Autodesk Inventor part; units mm, degrees
ref_plane "YZ Plane" through (0, 0, 0) normal (1, 0, 0) x (0, 1, 0)
ref_plane "XZ Plane" through (0, 0, 0) normal (0, 1, 0) x (-1, 0, 0)
ref_plane "XY Plane" through (0, 0, 0) normal (0, 0, 1) x (1, 0, 0)
sketch "Sketch1" plane through (0, 0, 0) normal (0, 0, 1) x (1, 0, 0)
  line L0 (0, 0) -> (0, -57.15) construction
  line L1 (0, 0) -> (-53.8815, -53.8815) construction
  line L2 (12.7, 3.175) -> (-14.7855, 3.175)
  line L3 (-14.7855, 3.175) -> (-62.8618, -44.9013)
  line L4 (-62.8618, -44.9013) -> (-44.9013, -62.8618)
  line L5 (-44.9013, -62.8618) -> (-12.7, -30.6605)
  line L6 (-12.7, -30.6605) -> (-12.7, -57.15)
  line L7 (-12.7, -57.15) -> (12.7, -57.15)
  line L8 (12.7, -57.15) -> (12.7, 3.175)
  dimension "d0" = 45
  dimension "d1" = 57.15
  dimension "d2" = 76.2
  dimension "d3" = 3.175
  dimension "d4" = 25.4
  dimension "d5" = 25.4
extrude "Extrusion1" add sketch "Sketch1" against normal blind 6.35
sketch "Sketch2" plane through (0, 0, 0) normal (0, 0, 1) x (1, 0, 0)
  line L0 (-44.9013, -62.8618) -> (-62.8618, -44.9013) construction
  line L1 (-62.8618, -44.9013) -> (-14.7855, 3.175) construction
  line L2 (-14.7855, 3.175) -> (12.7, 3.175) construction
  line L3 (12.7, 3.175) -> (12.7, -57.15) construction
  line L4 (12.7, -57.15) -> (-12.7, -57.15) construction
  line L5 (-12.7, -57.15) -> (-12.7, -30.6605) construction
  line L6 (-12.7, -30.6605) -> (-44.9013, -62.8618) construction
  line L7 (-44.9013, -62.8618) -> (-62.8618, -44.9013) construction
  line L8 (-62.8618, -44.9013) -> (-14.7855, 3.175) construction
  line L9 (-14.7855, 3.175) -> (12.7, 3.175) construction
  line L10 (12.7, 3.175) -> (12.7, -57.15) construction
  line L11 (12.7, -57.15) -> (-12.7, -57.15) construction
  line L12 (-12.7, -57.15) -> (-12.7, -30.6605) construction
  line L13 (-12.7, -30.6605) -> (-44.9013, -62.8618) construction
  line L14 (0, 0) -> (0, -57.15) construction
  line L15 (12.7, -57.15) -> (-12.7, -57.15) construction
  line L16 (0, 0) -> (-53.8815, -53.8815) construction
  line L17 (-44.9013, -62.8618) -> (-62.8618, -44.9013) construction
  line L18 (-12.7, -30.6605) -> (-12.7, 3.175) construction
  line L19 (-14.7855, 3.175) -> (12.7, 3.175) construction
  point P0 (-30.6605, -30.6605)
  point P1 (-48.621, -48.621)
  point P2 (0, -9.525)
  point P3 (0, -34.925)
  point P4 (-12.7, -12.7)
  point P5 (-12.7, -13.7428)
  dimension "d8" = 25.4
  dimension "d9" = 25.4
  dimension "d19" = 12.7
  dimension "d21" = 25.4
hole "Hole1" at (-30.6605, -30.6605, 0) at (-48.621, -48.621, 0) at (0, -9.525, 0) at (0, -34.925, 0) direction (0, 0, -1) diameter 5.1054 end through all
fillet "Fillet1" radius 6.35 7 edges at (12.7, 3.175, -3.175) (-14.7855, 3.175, -3.175) (-62.8618, -44.9013, -3.175) (-44.9013, -62.8618, -3.175) (-12.7, -30.6605, -3.175) (-12.7, -57.15, -3.175) (12.7, -57.15, -3.175)
equation "\"d5\" = d4"
properties part number "CL4-008" material "Aluminum 6061"
Part model, mm, in its own coordinate system. A direction names the side the tool comes from. Round coordinates to 2 decimals unless told otherwise and drop trailing zeros. Loops run counter-clockwise (first coordinate to the right, second up) from the corner with the lowest first, then second, coordinate; pieces in that order, holes last.
Item 1: 3-axis set-ups, long thin cutter, end or side, ignore diameter. For faces 1 (the face through (-16, -28, -6.35)), 2 (the face through (-10.79, -55.34, -3.22)): which of +Z, -Z, +X, -X, +Y, -Y reach the whole face in a straight line?
Item 2: Cut at A-A, the plane x = 0. Give the cut face in (y, z) (3 decimals), then the cut area to 3 significant figures.
Item 3: Cut at D-D, the plane y = -38.5. Give the cut face in (x, z).
Item 4: Cut at C-C, the plane x = -42. Give the cut face in (y, z), then the cut area to 3 significant figures.
Item 5: Cut at B-B, the plane z = -4. State how many separate pieces and enclosed holes the cut face has, then the cut area to 3 significant figures.
Item 6: Mould opens along Y. For faces 3 (the face through (-16, -28, 0)), 4 (the face through (-28.396, -31.838, -3.219)), 5 (the face through (0, -57.15, -3)) say: +Y half, -Y half, draft (parallel to the pull), parting line (faces both ways), or undercut.
Item 7: Drill centre lines: line 1 (Y direction, x = 0, z = -3.5) (3 decimals); line 2 (Y direction, x = -6.5, z = -4) (3 decimals); line 3 (X direction, y = -8.5, z = -1.75). Where is each one in solid material? Low to high.
Item 8: Drop a flat-ended pin along its axis: P1, Ø3, axis at y = -53.5, z = -1.5, coming from the -X side. Give the stop position or say it passes through.
A:
1. face 1: -Z, +X, -X, +Y, -Y
1. face 2: +Z, -Z, -Y
2. outline: (-57.15, -6.35) - (-37.478, -6.35) - (-37.478, 0) - (-57.15, 0) - close; (-32.372, -6.35) - (-12.078, -6.35) - (-12.078, 0) - (-32.372, 0) - close; (-6.972, -6.35) - (3.175, -6.35) - (3.175, 0) - (-6.972, 0) - close
2. area: 318 mm2
3. outline: (-56.46, -6.35) - (12.7, -6.35) - (12.7, 0) - (-56.46, 0) - close
4. outline: (-59.53, -6.35) - (-24.04, -6.35) - (-24.04, 0) - (-59.53, 0) - close
4. area: 225 mm2
5. separate pieces: 1
5. enclosed holes: 4
5. area: 2,930 mm2
6. face 3: draft
6. face 4: undercut
6. face 5: -Y half
7. line 1: y = -57.15 to -37.478, -32.372 to -12.078, -6.972 to 3.175
7. line 2: y = -57.148 to 3.175
7. line 3: x = -26.46 to -2.34, 2.34 to 12.7
8. P1: stops at x = -55.76
